Autodesk Inventor part; units mm, degrees
ref_plane "YZ Plane" through (0, 0, 0) normal (1, 0, 0) x (0, 1, 0)
ref_plane "XZ Plane" through (0, 0, 0) normal (0, 1, 0) x (-1, 0, 0)
ref_plane "XY Plane" through (0, 0, 0) normal (0, 0, 1) x (1, 0, 0)
sketch "スケッチ1" plane through (0, 0, 0) normal (0, 0, 1) x (1, 0, 0)
  line L0 (-14.75, -12.5) -> (14.75, -12.5)
  line L1 (14.75, -12.5) -> (14.75, 12.5)
  line L2 (14.75, 12.5) -> (-14.75, 12.5)
  line L3 (-14.75, 12.5) -> (-14.75, -12.5)
  line L4 (-14.75, -12.5) -> (14.75, 12.5) construction
  line L5 (14.75, -12.5) -> (-14.75, 12.5) construction
  point P0 (0, 0)
  dimension "d0" = 29.5
  dimension "d1" = 25
extrude "プレート1" add sketch "スケッチ1" along normal blind 5
sketch "スケッチ2" plane through (0, 0, 5) normal (0, 0, 1) x (1, 0, 0)
  line L0 (-12.25, -10.25) -> (8.75, -10.25) construction
  line L1 (8.75, -10.25) -> (8.75, 10.25) construction
  line L2 (8.75, 10.25) -> (-12.25, 10.25) construction
  line L3 (-12.25, 10.25) -> (-12.25, -10.25) construction
  line L4 (-12.25, -10.25) -> (8.75, 10.25) construction
  line L5 (8.75, -10.25) -> (-12.25, 10.25) construction
  line L6 (14.75, 12.5) -> (14.75, -12.5) construction
  point P0 (0, 0)
  point P1 (-1.75, 0)
  dimension "d3" = 21
  dimension "d4" = 20.5
  dimension "d5" = 6
hole "穴1" at (-12.25, 10.25, 5) at (8.75, 10.25, 5) at (8.75, -10.25, 5) at (-12.25, -10.25, 5) direction (0, 0, -1) diameter 2.1 end through all
sketch "スケッチ3" plane through (0, 0, 0) normal (0, 0, -1) x (-1, 0, 0)
  line L0 (-14.75, -12.5) -> (-14.75, 12.5)
  line L1 (14.75, 12.5) -> (14.75, -12.5)
  line L2 (-14.75, 7.7) -> (14.75, 7.7)
  line L3 (14.75, -7.7) -> (-14.75, -7.7)
  line L4 (-14.75, 12.5) -> (14.75, 12.5)
  line L5 (14.75, -12.5) -> (-14.75, -12.5)
  point P0 (0, 0)
  dimension "d13" = 4.8
  dimension "d14" = 4.8
extrude "押し出し1" cut sketch "スケッチ3" against normal blind 1.5 contours L0 L2 L1 L3
sketch "スケッチ4" plane through (0, 0, 5) normal (0, 0, 1) x (1, 0, 0)
  line L0 (-14.75, 12.5) -> (14.75, 12.5)
  line L1 (14.75, -12.5) -> (-14.75, -12.5)
  circle A0 centre (-20.25, 0) radius 11.5
  line L2 (14.75, 12.5) -> (14.75, -12.5)
  line L3 (-9.25, -9.6) -> (-9.25, 9.6)
  line L4 (9.75, 9.6) -> (9.75, -9.6)
  line L5 (9.75, -9.6) -> (-9.25, 9.6) construction
  line L6 (-9.25, -9.6) -> (9.75, 9.6) construction
  line L7 (-9.25, 7.7) -> (-11.7083, 7.7)
  line L8 (-11.7083, 7.7) -> (-11.7083, -7.7)
  line L9 (-11.7083, -7.7) -> (-9.25, -7.7)
  line L10 (-9.25, -7.7) -> (-9.25, 7.7)
  line L11 (14.75, 7.7) -> (-14.75, 7.7)
  line L12 (14.75, 7.7) -> (-14.75, 7.7)
  line L13 (14.75, 7.7) -> (-14.75, 7.7)
  line L14 (-14.75, -7.7) -> (14.75, -7.7)
  line L15 (-14.75, -7.7) -> (14.75, -7.7)
  point P0 (0, 0)
  point P1 (14.75, 0)
  point P2 (0.25, 0)
  point P3 (-9.25, 0)
  point P4 (-11.7083, 7.7)
  point P5 (-9.25, -3.3541)
  point P6 (-9.25, 3.3541)
  point P7 (9.75, -7.7)
  point P8 (9.75, 7.7)
  dimension "d18" = 23
  dimension "d17" = 35
  dimension "d19" = 5
  dimension "d22" = 19
extrude "押し出し2" cut sketch "スケッチ4" against normal through all contours L8 A0 | L7 L3 A0 | A0 L3 L8 | A0 L3 L9 | L3 L11 L4 L14 A0 | A0 L3
fillet "フィレット1" radius 1 10 edges at (-11.7083, -7.7, 2.5) (-11.7083, 7.7, 2.5) (-14.75, -10.0995, 2.5) (-14.75, 10.0995, 2.5) (-14.75, -12.5, 2.5) (14.75, -12.5, 2.5) (14.75, 12.5, 2.5) (-14.75, 12.5, 2.5) (9.75, 7.7, 3.25) (9.75, -7.7, 3.25)
sketch "スケッチ5" plane through (0, 0, 5) normal (0, 0, 1) x (1, 0, 0)
  line L0 (-13.75, 12.5) -> (13.75, 12.5)
  circle A0 centre (-7.25, 13.4) radius 1.05
  circle A1 centre (4.75, 13.4) radius 1.05
  line L1 (14.75, 11.5) -> (14.75, -11.5)
  point P0 (0, 0)
  point P1 (-14.75, 12.5)
  point P2 (14.75, 12.5)
  point P3 (14.75, -12.5)
  dimension "d26" = 2.1
  dimension "d27" = 2.1
  dimension "d28" = 0.9
  dimension "d29" = 0.9
  dimension "d30" = 12
  dimension "d31" = 10
extrude "押し出し3" cut sketch "スケッチ5" against normal through all
sketch "スケッチ6" plane through (-6.7092, 12.5, 0) normal (0, 1, 0) x (1, 0, 0)
  line L0 (-1.0817, -5) -> (-1.0817, 0)
  line L1 (0, -5) -> (-1.0817, -5)
  line L2 (0, 0) -> (0, -5)
  line L3 (-1.0817, 0) -> (0, 0)
  line L4 (10.9183, -5) -> (10.9183, 0)
  line L5 (12, -5) -> (10.9183, -5)
  line L6 (12, 0) -> (12, -5)
  line L7 (10.9183, 0) -> (12, 0)
  line L8 (-1.5408, -3) -> (-1.5408, 0) construction
  line L9 (-1.5408, 0) -> (-1.5408, -3) construction
  line L10 (-1.0817, -2.5) -> (0, -2.5) construction
  line L11 (10.9183, -2.5) -> (12, -2.5) construction
  line L12 (11.4592, -5) -> (11.4592, 0) construction
  point P0 (6.7092, 0)
  point P1 (-0.5408, -2.5)
  point P2 (11.4592, -2.5)
hole "穴2" at (-7.25, 12.5, 2.5) at (4.75, 12.5, 2.5) direction (0, -1, 0) diameter 2.5 end through all
mirror "ミラー1" about plane through (0, 0, 0) normal (0, 1, 0) of "穴2", "押し出し3"
equation "\"d11\" = Thickness"
equation "\"d14\" = d13"
equation "\"d29\" = d28"
equation "\"d2\" = Thickness"
equation "\"BendRadius\" = Thickness"
equation "\"BendReliefWidth\" = Thickness"
equation "\"BendReliefDepth\" = 0.5 * Thickness"
equation "\"TransitionRadius\" = BendRadius"
equation "\"JacobiRadiusSize\" = BendRadius"
equation "\"GapSize\" = Thickness"
properties part number "T3.0_servo-mount_bottom_3D プリント"
Input: part model. Units: mm. Frame: model coordinates. A direction names the side the tool comes from. Give positions to 0.01 mm unless a question says otherwise; leave off trailing zeros. Order: outer loops, then holes, each group sorted by start corner. A loop starts at its lowest first (then second) coordinate and runs counter-clockwise, first axis right, second up. Notation, with made-up numbers: M 24.5,66 L 47.5,66 A16 ccw 47.5,89 Z; hole C 48,-36 d6. An arc over 180 degrees is marked long. Return JSON: item names as keys, results as strings.
Item 1: Pull-direction query (Y, two-part tool) for faces 3 (the flat face through (3, 9, 5)), 4 (the cylindrical face through (-14.449, 12.215, 2.535)), 5 (the cylindrical face through (-13.057, 8.973, 2.535)); classes: +Y half, -Y half, draft (parallel to the pull), parting line (faces both ways), or undercut.
Solutions:
{"face 3": "draft", "face 4": "+Y half", "face 5": "undercut"}
Item 2: Access query for faces 1 (the cylindrical face through (9.449, 7.415, 3.226)), 2 (the cylindrical face through (14.465, 12.199, 2.535)). Directions: +Z, -Z, +X, -X, +Y, -Y. A direction counts if a zero-diameter tool reaches every point of the face in a straight line with its end or side. Return the directions, or none.
Solutions:
{"face 1": "+Z, -Z, -X", "face 2": "+Z, -Z, +X, +Y"}
Item 3: Cut plane D-D (x = -7.25). Return loops of the section in (y, z), then the cut area to 4 significant figures.
Solutions:
{"outline": "M -12.35,0 L -7.7,0 L -7.7,1.25 L -12.35,1.25 Z; M -12.35,3.75 L -7.7,3.75 L -7.7,5 L -12.35,5 Z; M 7.7,0 L 12.35,0 L 12.35,1.25 L 7.7,1.25 Z; M 7.7,3.75 L 12.35,3.75 L 12.35,5 L 7.7,5 Z", "area": "23.25 mm^2"}
Item 4: Cut plane C-C (y = -10.25). Return loops of the section in (x, z).
Solutions:
{"outline": "M -14.65,0 L -13.3,0 L -13.3,5 L -14.65,5 Z; M -11.2,0 L 7.7,0 L 7.7,5 L -11.2,5 Z; M 9.8,0 L 14.75,0 L 14.75,5 L 9.8,5 Z; hole C -7.25,2.5 d2.5; hole C 4.75,2.5 d2.5"}
Item 5: Ray query, probe 1 along Z at (x, y) = (-7.25, 11.55); probe 2 along Z at (x, y) = (4, -10.75); probe 3 along Y at (x, z) = (8.75, 2.2). Return the intervals inside material, ascending.
Solutions:
{"probe 1": "0 to 1.25, 3.75 to 5", "probe 2": "0 to 1.5, 3.5 to 5", "probe 3": "-12.5 to -11.3, -9.2 to -7.7, 7.7 to 9.2, 11.3 to 12.5"}
Item 6: First-contact query: P1, Ø3, axis at x = 11, y = 1.5, coming from the -Z side; P2, Ø1.8, axis at y = -0.5, z = 3.5, coming from the -X side. Flat tips, straight axial feed; report the tip coordinate or a pass-through.
Solutions:
{"P1": "z = 1.5", "P2": "x = 9.75"}
Item 7: Cut plane A-A (z = 0.45). State how many separate pieces and enclosed holes the cut face has, then the cut area to 3 significant figures.
Solutions:
{"separate pieces": "2", "enclosed holes": "4", "area": "260 mm^2"}
Item 8: Cut plane B-B (x = 1). Return loops of the section in (y, z), then the cut area to 3 significant figures.
Solutions:
{"outline": "M -12.5,0 L -7.7,0 L -7.7,5 L -12.5,5 Z; M 7.7,0 L 12.5,0 L 12.5,5 L 7.7,5 Z", "area": "48.0 mm^2"}
